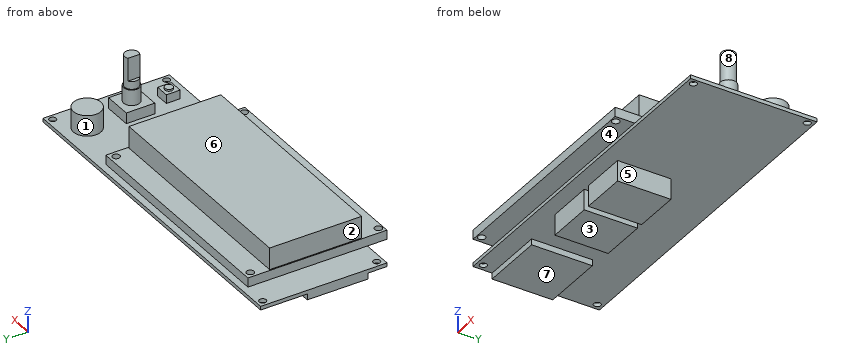
```python
from build123d import *

# Parameters (mm, degrees)
SKETCH1_W                          = 150.0378
SKETCH1_H                          = 54.991
BOSS_EXTRUDE1_DEPTH                = 1.6002
SKETCH2_W                          = 98
SKETCH2_H                          = 60.5
BOSS_EXTRUDE2_DEPTH                = 4
SKETCH3_W                          = 97
SKETCH3_H                          = 40
BOSS_EXTRUDE3_DEPTH                = 9.5
SKETCH4_R                          = 6
BOSS_EXTRUDE4_DEPTH                = 9
SKETCH5_W                          = 12.2
SKETCH5_H                          = 12.4
BOSS_EXTRUDE5_DEPTH                = 4.7
SKETCH6_R                          = 3.5
BOSS_EXTRUDE6_DEPTH                = 6.8
SKETCH7_R                          = 3
BOSS_EXTRUDE7_DEPTH                = 13.4
SKETCH8_W                          = 1.5
SKETCH8_H                          = 5.196152422
CUT_EXTRUDE1_DEPTH                 = 10
SKETCH9_W                          = 6
SKETCH9_H                          = 6
BOSS_EXTRUDE8_DEPTH                = 3.8
SKETCH10_R                         = 1.75
BOSS_EXTRUDE9_DEPTH                = 0.8
SKETCH11_W                         = 27.3
SKETCH11_H                         = 26.4
BOSS_EXTRUDE10_DEPTH               = 2.6
SKETCH12_W                         = 20.2
SKETCH12_H                         = 23.2
BOSS_EXTRUDE11_DEPTH               = 9
F_3_0_3_DIAMETER_HOLE1_D           = 3
F_3_2_START                        = 1.6002
F_3_2_3_2_DIAMETER_HOLE1_OUTLINE_R = 1.6
F_3_2_3_2_DIAMETER_HOLE1_DEPTH     = 4


# Read off the part's stored shape, not the designer's step: Ø3.2 (3.2) Diameter Hole1
with BuildPart() as part:
    # Sketch1 → Boss-Extrude1 (new body)
    with BuildSketch(Plane.XY):
        Rectangle(SKETCH1_W, SKETCH1_H)
    extrude(amount=BOSS_EXTRUDE1_DEPTH)

    # Sketch2 → Boss-Extrude2 (add)
    with BuildSketch(Plane.XY.offset(1.6002)):
        with Locations((-12.5189, -5.7545)):
            Rectangle(SKETCH2_W, SKETCH2_H)
    extrude(amount=BOSS_EXTRUDE2_DEPTH)

    # Sketch3 → Boss-Extrude3 (add)
    with BuildSketch(Plane.XY.offset(5.6002)):
        with Locations((-12.5189, -5.2545)):
            Rectangle(SKETCH3_W, SKETCH3_H)
    extrude(amount=BOSS_EXTRUDE3_DEPTH)

    # Sketch4 → Boss-Extrude4 (add)
    with BuildSketch(Plane.XY.offset(1.6002)):
        with Locations(Location((61.2189, 16.9955, 0), (0, 0, 180))):
            Circle(SKETCH4_R)
    extrude(amount=BOSS_EXTRUDE4_DEPTH)

    # Sketch5 → Boss-Extrude5 (add)
    with BuildSketch(Plane.XY.offset(1.6002)):
        with Locations((61.7189, -2.6955)):
            Rectangle(SKETCH5_W, SKETCH5_H)
    extrude(amount=BOSS_EXTRUDE5_DEPTH)

    # Sketch6 → Boss-Extrude6 (add)
    with BuildSketch(Plane.XY.offset(6.3002)):
        with Locations((61.7189, -2.6955)):
            Circle(SKETCH6_R)
    extrude(amount=BOSS_EXTRUDE6_DEPTH)

    # Sketch7 → Boss-Extrude7 (add)
    with BuildSketch(Plane.XY.offset(13.1002)):
        with Locations((61.7189, -2.6955)):
            Circle(SKETCH7_R)
    extrude(amount=BOSS_EXTRUDE7_DEPTH)

    # Sketch8 → Cut-Extrude1 (cut)
    with BuildSketch(Plane.XY.offset(26.5002)):
        with Locations((59.4689, -2.6955)):
            Rectangle(SKETCH8_W, SKETCH8_H)
    extrude(amount=-CUT_EXTRUDE1_DEPTH, mode=Mode.SUBTRACT)

    # Sketch9 → Boss-Extrude8 (add)
    with BuildSketch(Plane.XY.offset(1.6002)):
        with Locations((62.2689, -19.2455)):
            Rectangle(SKETCH9_W, SKETCH9_H)
    extrude(amount=BOSS_EXTRUDE8_DEPTH)

    # Sketch10 → Boss-Extrude9 (add)
    with BuildSketch(Plane.XY.offset(5.4002)):
        with Locations((62.2689, -19.2455)):
            Circle(SKETCH10_R)
    extrude(amount=BOSS_EXTRUDE9_DEPTH)

    # Sketch11 → Boss-Extrude10 (add)
    with BuildSketch(Plane(origin=(0, 0, 0), x_dir=(-1, 0, 0), z_dir=(0, 0, -1))):
        with Locations((61.3689, -5.9955)):
            Rectangle(SKETCH11_W, SKETCH11_H)
    extrude(amount=BOSS_EXTRUDE10_DEPTH)

    # Sketch12 → Boss-Extrude11 (add)
    with BuildSketch(Plane(origin=(0, 0, 0), x_dir=(-1, 0, 0), z_dir=(0, 0, -1))):
        with Locations((19.2189, -9.0955)):
            Rectangle(SKETCH12_W, SKETCH12_H)
        with Locations((-3.7811, -9.0955)):
            Rectangle(SKETCH12_W, SKETCH12_H)
    extrude(amount=BOSS_EXTRUDE11_DEPTH)

    # Ø3.0 (3) Diameter Hole1 (through all)
    with Locations(Plane.XY.offset(1.6002)):
        with Locations((-72.2689, 24.8455), (-72.2689, -24.7455), (72.5189, -24.7455), (72.5189, 24.8455)):
            Hole(F_3_0_3_DIAMETER_HOLE1_D / 2)

    # Ø3.2 (3.2) Diameter Hole1 outline → Ø3.2 (3.2) Diameter Hole1 (cut)
    with BuildSketch(Plane.XY.offset(F_3_2_START)):
        with Locations((-58.7689, -34.0045)):
            Circle(F_3_2_3_2_DIAMETER_HOLE1_OUTLINE_R)
        with Locations((33.7311, -34.0045)):
            Circle(F_3_2_3_2_DIAMETER_HOLE1_OUTLINE_R)
        with Locations((33.7311, 21.7455)):
            Circle(F_3_2_3_2_DIAMETER_HOLE1_OUTLINE_R)
        with Locations((-58.7689, 21.7455)):
            Circle(F_3_2_3_2_DIAMETER_HOLE1_OUTLINE_R)
    extrude(amount=F_3_2_3_2_DIAMETER_HOLE1_DEPTH, mode=Mode.SUBTRACT)


solid = part.part
```
Check sheet for the modelled part. Datum: model origin and axes. Units: mm. Face numbers are marked on the shaded views. A direction names the side the tool comes from. Coordinates: 2 decimals unless noted, no trailing zeros. Order: outer loops, then holes, each group sorted by start corner. A loop starts at its lowest first (then second) coordinate and runs counter-clockwise, first axis right, second up. Notation, with made-up numbers: (-30, 62) -> (4, 62) arc R26 ccw to (4, 96) -> close; hole circle Ø2 at (14, -30). An arc over 180 degrees is marked (long way). Write each question's results on one line, items separated by ' | '. Start each with the question number.
1) Draft check along X on the marked faces 1, 2 and 3. Enter one of: pulls with the +X half, pulls with the -X half, needs draft (parallel to the pull), parting line crosses it, or undercut.
2) Section check B-B (z = 8). Enter the section's corners in (x, y).
3) Section check D-D (x = 46.5). Enter the section's corners in (y, z).
4) Section check C-C (z = 23.5). Enter the section's corners in (x, y), and give its area (3 significant figures).
5) Depth check by flat-ended pin: pin 1 (2 mm diameter, centred on x = -19, z = 3.5, fed in from +Y); pin 2 (10 mm diameter, centred on x = 29.5, y = -12, fed in from +Z); pin 3 (6 mm diameter, centred on y = 20, z = 12, fed in from -X); pin 4 (2.5 mm diameter, centred on x = 72.52, y = 24.85, fed in from -Z). Enter the tip coordinate at first touch or a pass-through.
6) Set-up check for the marked faces 4, 5, 6, 7 and 8: record each of +Z, -Z, +X, -X, +Y, -Y from which the full face is reachable in a straight line by a thin tool's end or side.
7) Material ranges on line 1 along X through (y, z) = (16.5, 4); line 2 along X through (y, z) = (-20.5, -7); line 3 along Y through (x, z) = (-60, 5), recorded low to high.
8) Section check A-A (x = -21.5). Enter the section's corners in (y, z), and give its area (3 significant figures).
Checked values:
1) face 1: undercut | face 2: pulls with the -X half | face 3: needs draft
2) outline: (-61.02, -25.25) -> (35.98, -25.25) -> (35.98, 14.75) -> (-61.02, 14.75) -> close; circle Ø12 at (61.22, 17); circle Ø7 at (61.72, -2.7)
3) outline: (-27.5, 0) -> (27.5, 0) -> (27.5, 1.6) -> (-27.5, 1.6) -> close
4) outline: (60.22, -5.29) arc R3 ccw (long way) to (60.22, -0.1) -> close | area: 22.7 mm²
5) pin 1: y = 24.5 | pin 2: z = 15.1 | pin 3: x = 55.23 | pin 4: through
6) face 4: -Z, +X, -X, -Y | face 5: -Z, +X, +Y, -Y | face 6: +Z, -X, +Y, -Y | face 7: -Z, -X, +Y, -Y | face 8: +Z
7) line 1: -61.52 to 36.48, 55.24 to 67.2 | line 2: -29.32 to -9.12, -6.32 to 13.88 | line 3: -36 to -35.03, -32.98 to 20.72, 22.77 to 24.5
8) outline: (-36, 1.6) -> (-27.5, 1.6) -> (-27.5, 0) -> (-20.7, 0) -> (-20.7, -9) -> (2.5, -9) -> (2.5, 0) -> (27.5, 0) -> (27.5, 1.6) -> (24.5, 1.6) -> (24.5, 5.6) -> (14.75, 5.6) -> (14.75, 15.1) -> (-25.25, 15.1) -> (-25.25, 5.6) -> (-36, 5.6) -> close | area: 919 mm²
